Read the model definition and answer for the solid it produces. Units are mm, in the model's axes. Face numbers are marked on the shaded views. A direction names the side the tool comes from. Coordinates: 2 decimals unless noted, no trailing zeros. Write each loop counter-clockwise with the first axis right and the second up, starting at its lowest first coordinate (ties: lowest second). Pieces come first, ordered by that corner, then holes.
1) Each of these flat-tipped pins is pushed along its axis until it touches: pin 1 Ø1 at (y, z) = (5.5, -3) entering from +X; pin 2 Ø2 at (x, z) = (5, -0.5) entering from -Y. Where does it stop, or does it pass through?
2) Determine the mould class of the marked faces 3, 4 and 5 for opening direction Y: +Y half, -Y half, draft (parallel to the pull), parting line (faces both ways), or undercut.
3) Which of the six approach directions +Z, -Z, +X, -X, +Y, -Y give full straight-line access (tool end or side, diameter ignored) to the marked faces 1 and 2?
4) The part is cut by section C-C (y = 0.75). Determine the outline of the cut face in (x, z).
5) The part is cut by section B-B (z = -4.35). Determine the outline of the cut face in (x, y).
6) Find the intervals of material crossed by line 1 (X direction, y = 0.25, z = -0.25); line 2 (X direction, y = -1.75, z = -1.8); line 3 (Y direction, x = 3, z = -1.1), in increasing order.
7) The part is cut by section D-D (x = 4.5). Determine the outline of the cut face in (y, z), then the cut area to 3 significant figures.
8) The part is cut by section A-A (x = 0). Determine the outline of the cut face in (y, z).
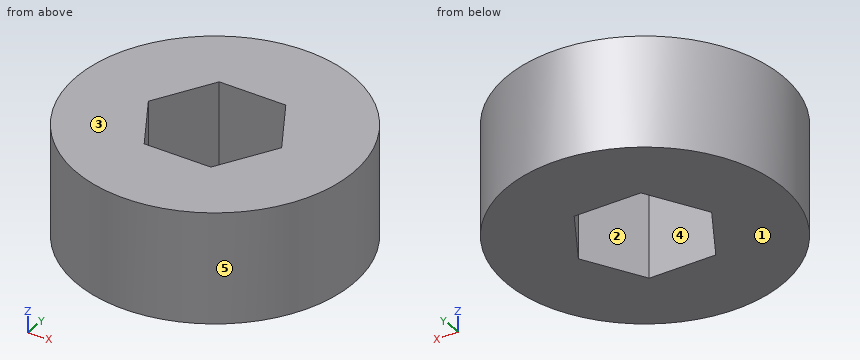
Autodesk Inventor part; units mm, degrees
ref_plane "YZ Plane" through (0, 0, 0) normal (1, 0, 0) x (0, 1, 0)
ref_plane "XZ Plane" through (0, 0, 0) normal (0, 1, 0) x (-1, 0, 0)
ref_plane "XY Plane" through (0, 0, 0) normal (0, 0, 1) x (1, 0, 0)
sketch "Sketch1" plane through (0, 0, 0) normal (0, 0, 1) x (1, 0, 0)
  line L0 (-1.6732, 2.8981) -> (1.6732, 2.8981)
  line L1 (-3.3464, 0) -> (-1.6732, 2.8981)
  line L2 (-1.6732, -2.8981) -> (-3.3464, 0)
  line L3 (1.6732, -2.8981) -> (-1.6732, -2.8981)
  line L4 (3.3464, 0) -> (1.6732, -2.8981)
  line L5 (1.6732, 2.8981) -> (3.3464, 0)
  circle A0 centre (0, 0) radius 7.5
extrude "Extrusion1" add sketch "Sketch1" against normal blind 6
sketch "Sketch2" plane through (0, 0, 0) normal (0, 0, 1) x (1, 0, 0)
  circle A0 centre (0, 0) radius 7.5
  line L0 (0, 0) -> (-3.1, 0) construction
  line L1 (0, 0) -> (-1.55, -2.6847) construction
  line L2 (0, 0) -> (1.55, -2.6847) construction
  line L3 (0, 0) -> (3.1, 0) construction
  line L4 (0, 0) -> (1.55, 2.6847) construction
  line L5 (0, 0) -> (-1.55, 2.6847) construction
  line L6 (1.55, 2.6847) -> (-1.55, 2.6847) construction
  line L7 (1.6732, 2.8981) -> (-1.6732, 2.8981)
  line L8 (-1.55, 2.6847) -> (-3.1, 0) construction
  line L9 (1.55, -2.6847) -> (-1.55, -2.6847) construction
  line L10 (-1.6732, -2.8981) -> (1.6732, -2.8981)
  line L11 (-1.55, -2.6847) -> (-3.1, 0) construction
  line L12 (1.55, -2.6847) -> (3.1, 0) construction
  line L13 (3.1, 0) -> (1.55, 2.6847) construction
  line L14 (3.3464, 0) -> (1.6732, 2.8981)
  line L15 (-1.8098, 3.1347) -> (1.8098, 3.1347)
  line L16 (1.8098, 3.1347) -> (3.6196, 0)
  line L17 (3.6196, 0) -> (1.8098, -3.1347)
  line L18 (1.8098, -3.1347) -> (-1.8098, -3.1347)
  line L19 (-1.8098, -3.1347) -> (-3.6196, 0)
  line L20 (-3.6196, 0) -> (-1.8098, 3.1347)
  point P0 (0, 0)
  dimension "d4" = 3.1
  dimension "d7" = 360
  dimension "d9" = 0.45
extrude "Extrusion2" cut sketch "Sketch2" against normal blind 10 contours L15 L16 L17 L18 L19 L20
properties part number "Rodamiento_Ejes"
Reported:
1. pin 1: stops at x = 5.59
1. pin 2: stops at y = -6.34
2. face 3: draft
2. face 4: undercut
2. face 5: parting line
3. face 1: -Z, +X, -X, +Y, -Y
3. face 2: +Z, -Z
4. outline: (-7.46, -6) - (-3.19, -6) - (-3.19, 0) - (-7.46, 0) - close; (3.19, -6) - (7.46, -6) - (7.46, 0) - (3.19, 0) - close
5. outline: circle Ø15 at (0, 0); hole (-3.62, 0) - (-1.81, -3.13) - (1.81, -3.13) - (3.62, 0) - (1.81, 3.13) - (-1.81, 3.13) - close
6. line 1: x = -7.5 to -3.48, 3.48 to 7.5
6. line 2: x = -7.29 to -2.61, 2.61 to 7.29
6. line 3: y = -6.87 to -1.07, 1.07 to 6.87
7. outline: (-6, -6) - (6, -6) - (6, 0) - (-6, 0) - close
7. area: 72.0 mm2
8. outline: (-7.5, -6) - (-3.13, -6) - (-3.13, 0) - (-7.5, 0) - close; (3.13, -6) - (7.5, -6) - (7.5, 0) - (3.13, 0) - close
